from build123d import *

# Parameters (mm, degrees)
BOSS_EXTRUDE1_DEPTH = 1.524


with BuildPart() as part:
    # Sketch1 → Boss-Extrude1 (new body)
    with BuildSketch(Plane.XY):
        with BuildLine():
            Line((0, 114.851197301), (1.524, 114.851197301))
            Line((1.524, 114.851197301), (1.524, 127.137521288))
            ThreePointArc((1.524, 127.137521288), (5.925149422, 122.754651777), (7.476746905, 116.740318344))
            ThreePointArc((7.476746905, 116.740318344), (7.739144324, 113.314611295), (10.032707403, 110.756508563))
            ThreePointArc((10.032707403, 110.756508563), (8.763036176, 109.151405897), (8.701919017, 107.105755809))
            ThreePointArc((8.701919017, 107.105755809), (8.227293035, 106.400067512), (7.656654449, 105.769482545))
            Line((7.656654449, 105.769482545), (5.742583542, 109.386323923))
            Line((5.742583542, 109.386323923), (4.395578742, 108.673474663))
            Line((4.395578742, 108.673474663), (6.414912826, 104.857727272))
            ThreePointArc((6.414912826, 104.857727272), (4.010280896, 104.139935188), (1.524, 104.480357725))
            Line((1.524, 104.480357725), (0, 104.480357725))
            ThreePointArc((0, 104.480357725), (-2.486280896, 104.139935188), (-4.890912826, 104.857727272))
            Line((-4.890912826, 104.857727272), (-2.871578742, 108.673474663))
            Line((-2.871578742, 108.673474663), (-4.218583542, 109.386323923))
            Line((-4.218583542, 109.386323923), (-6.132654449, 105.769482545))
            ThreePointArc((-6.132654449, 105.769482545), (-6.703293035, 106.400067512), (-7.177919017, 107.105755809))
            ThreePointArc((-7.177919017, 107.105755809), (-7.239036176, 109.151405897), (-8.508707403, 110.756508563))
            ThreePointArc((-8.508707403, 110.756508563), (-6.215144324, 113.314611295), (-5.952746905, 116.740318344))
            ThreePointArc((-5.952746905, 116.740318344), (-4.401149422, 122.754651777), (0, 127.137521288))
            Line((0, 127.137521288), (0, 114.851197301))
        make_face()
    extrude(amount=BOSS_EXTRUDE1_DEPTH)


solid = part.part
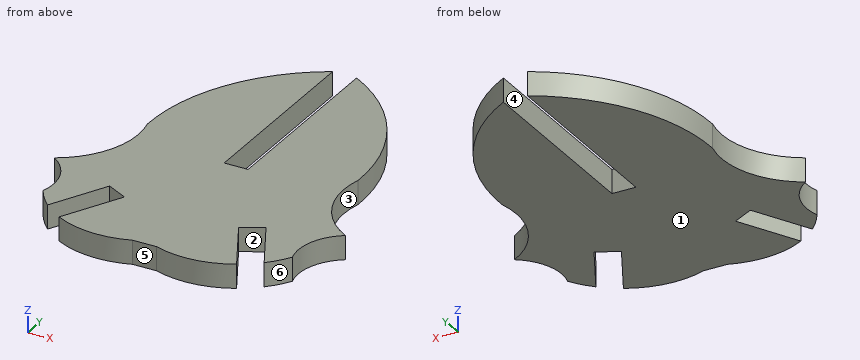
CAD build for the part. Positions are in the model's coordinates, mm. Face numbers are marked on the shaded views. A direction names the side the tool comes from. Round coordinates to 2 decimals unless told otherwise and drop trailing zeros. Write each loop counter-clockwise with the first axis right and the second up, starting at its lowest first coordinate (ties: lowest second). Pieces come first, ordered by that corner, then holes. Notation, with made-up numbers: M -39,57.5 L 2,57.5 A16 ccw 2,86.5 Z; hole C 75.5,87 d6. An arc over 180 degrees is marked long. Use a Markdown table: item, result. Add a question column.
1. Flat gauge pins, fed straight in: P1, Ø0.8, axis at x = 0.5, z = 0.5, coming from the -Y side; P2, Ø0.8, axis at x = 1, z = 1, coming from the +Y side. Where does each tip first touch, or does it go through?
2. Pull direction X, two halves, no side cores. Call the marked faces 1, 2 and 3: released by +X, released by -X, zero draft, split by the parting line, or undercut.
3. Slice it at D-D on x = 1. Give the cut face in (y, z), then the cut area to 3 significant figures.
4. 3-axis set-ups, long thin cutter, end or side, ignore diameter. For the marked faces 4, 5 and 6: which of +Z, -Z, +X, -X, +Y, -Y reach the whole face in a straight line?
5. Slice it at A-A on y = 125.25. Give the cut face in (x, z).
6. Slice it at C-C on z = 0.8. Give the cut face in (x, y), then the cut area to 3 significant figures.
7. Drill centre lines: probe 1 along X at (y, z) = (107.5, 0.25); probe 2 along X at (y, z) = (106.25, 0.6); probe 3 along Y at (x, z) = (0.5, 0.5). Where is each one in solid material? Low to high.
8. Slice it at B-B on y = 107.5. Give the cut face in (x, z), then the cut area to 3 significant figures.
Reply:
| question | item | result |
|---|---|---|
| 1 | P1 | stops at y = 104.48 |
| 1 | P2 | stops at y = 114.85 |
| 2 | face 1 | zero draft |
| 2 | face 2 | undercut |
| 2 | face 3 | released by +X |
| 3 | outline | M 104.48,0 L 114.85,0 L 114.85,1.52 L 104.48,1.52 Z |
| 3 | area | 15.8 mm^2 |
| 4 | face 4 | +Z, -Z, +Y |
| 4 | face 5 | +Z, -Z, -Y |
| 4 | face 6 | +Z, -Z, +X, -Y |
| 5 | outline | M -2.49,0 L 0,0 L 0,1.52 L -2.49,1.52 Z; M 1.52,0 L 4.01,0 L 4.01,1.52 L 1.52,1.52 Z |
| 6 | outline | M -8.51,110.76 A3.26 cw -7.18,107.11 A5.93 ccw -6.13,105.77 L -4.22,109.39 L -2.87,108.67 L -4.89,104.86 A5.93 ccw 0,104.48 L 1.52,104.48 A5.93 ccw 6.41,104.86 L 4.4,108.67 L 5.74,109.39 L 7.66,105.77 A5.93 ccw 8.7,107.11 A3.26 cw 10.03,110.76 A5.34 cw 7.48,116.74 A11.75 ccw 1.52,127.14 L 1.52,114.85 L 0,114.85 L 0,127.14 A11.75 ccw -5.95,116.74 A5.34 cw Z |
| 6 | area | 255 mm^2 |
| 7 | probe 1 | x = -7.09 to -5.22, -3.49 to 5.02, 6.74 to 8.61 |
| 7 | probe 2 | x = -6.58 to -5.88, -4.15 to 5.68, 7.4 to 8.11 |
| 7 | probe 3 | y = 104.48 to 114.85 |
| 8 | outline | M -7.09,0 L -5.22,0 L -5.22,1.52 L -7.09,1.52 Z; M -3.49,0 L 5.02,0 L 5.02,1.52 L -3.49,1.52 Z; M 6.74,0 L 8.61,0 L 8.61,1.52 L 6.74,1.52 Z |
| 8 | area | 18.7 mm^2 |
